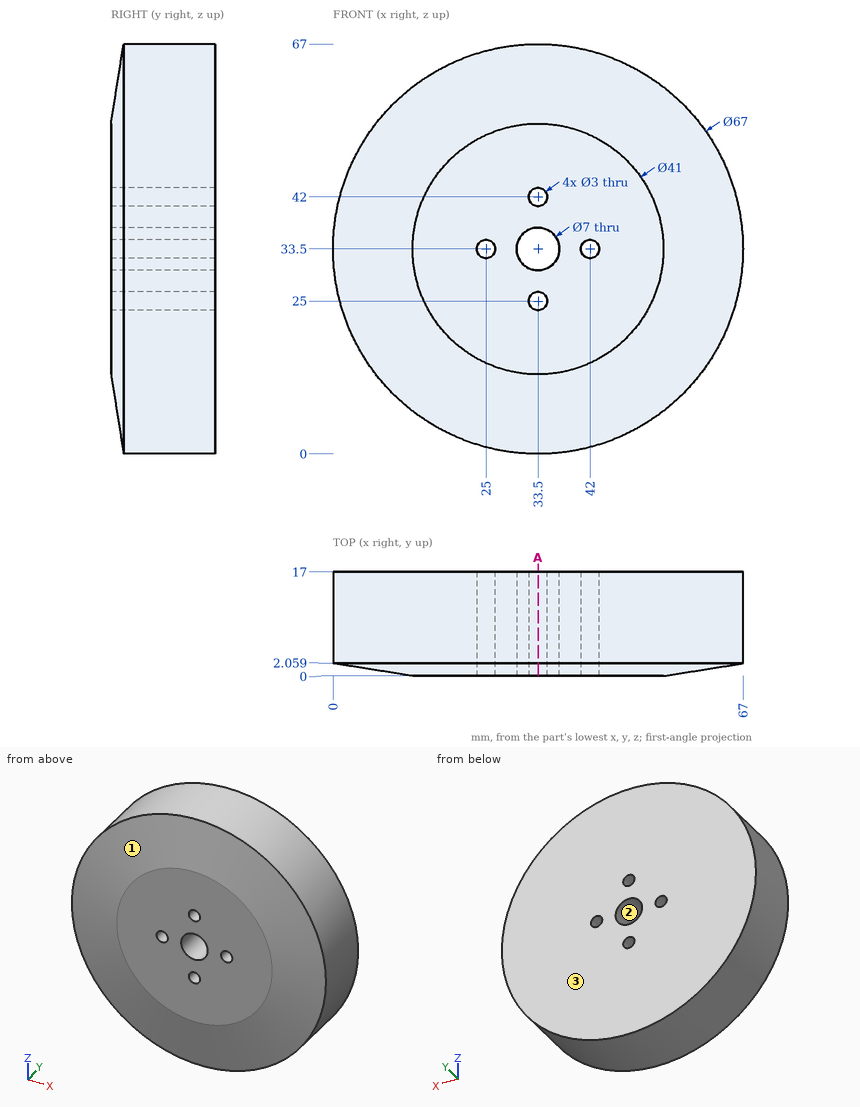
Here's the drawing with two shaded views (mm, measured from the low corner). I have some questions. Round coordinates to 2 decimals unless told otherwise and drop trailing zeros. Loops run counter-clockwise (first coordinate to the right, second up) from the corner with the lowest first, then second, coordinate; pieces in that order, holes last. Notation, with made-up numbers: (15.25, 26) - (65.25, 26) arc R23 cw to (65.25, 36) - close; hole circle Ø10 at (48, 37). An arc over 180 degrees is marked (long way). Use CSV: the item, a comma, the result in double quotes.
Item 1: I need wall thicknesses on L1, parallel to Z at x = 33.5, y = 4; L2, parallel to X at y = 13, z = 34.5. Which ranges of each line are inside material? Lowest first, please. Write a range as [from, to].
Here are the results:
L1,"z = [0, 23.5], [26.5, 30], [37, 40.5], [43.5, 67]"
L2,"x = [0.01, 23.88], [26.12, 30.15], [36.85, 40.88], [43.12, 66.99]"
Item 2: If we section it at A-A on x = 33.5: List the corners of the cut face in (y, z) for me.
Here are the results:
outline,"(0, 13) - (2.06, 0) - (17, 0) - (17, 23.5) - (0, 23.5) - close; (0, 26.5) - (17, 26.5) - (17, 30) - (0, 30) - close; (0, 37) - (17, 37) - (17, 40.5) - (0, 40.5) - close; (0, 43.5) - (17, 43.5) - (17, 67) - (2.06, 67) - (0, 54) - close"
Item 3: If we mould it in two halves opening along X, with no side actions, what happens to the marked faces 1, 2 and 3? For each: pulls with the +X half, pulls with the -X half, needs draft (parallel to the pull), parting line crosses it, or undercut.
Here are the results:
face 1,"parting line crosses it"
face 2,"undercut"
face 3,"needs draft"
Item 4: Will these pins go through, and if not, where does the flat tip stop? pin 1 (5 mm diameter, centred on x = 23.5, y = 15, fed in from -Z); pin 2 (2 mm diameter, centred on y = 10, z = 20, fed in from +X); pin 3 (5 mm diameter, centred on y = 10, z = 17, fed in from +X).
Here are the results:
pin 1,"stops at z = 0.85"
pin 2,"stops at x = 64.58"
pin 3,"stops at x = 63.93"
